```python
from build123d import *

# Parameters (mm, degrees)
SALIENTE_EXTRUIR2_DEPTH = 24
CROQUIS2_W              = 4.5
CROQUIS2_H              = 8
SALIENTE_EXTRUIR3_DEPTH = 24
CROQUIS3_W              = 7.5
CROQUIS3_H              = 3
SALIENTE_EXTRUIR4_DEPTH = 24
CORTAR_EXTRUIR1_START   = -8.720486
CROQUIS4_R              = 1.75
CORTAR_EXTRUIR1_DEPTH   = 17.440972
CROQUIS5_R              = 1.75
CORTAR_EXTRUIR2_DEPTH   = 10


with BuildPart() as part:
    # Croquis1 → Saliente-Extruir2 (new body)
    with BuildSketch(Plane.XY):
        with BuildLine():
            Line((-4.220485754, 10), (-12.5, 10))
            Line((-12.5, 10), (-12.5, -10))
            Line((-12.5, -10), (12.5, -10))
            Line((12.5, -10), (12.5, 10))
            Line((12.5, 10), (4.220485754, 10))
            ThreePointArc((4.220485754, 10), (0, -4.25), (-4.220485754, 10))
        make_face()
    extrude(amount=SALIENTE_EXTRUIR2_DEPTH)

    # Croquis2 → Saliente-Extruir3 (add)
    with BuildSketch(Plane.XY):
        with Locations((-6.470485754, 14)):
            Rectangle(CROQUIS2_W, CROQUIS2_H)
        with Locations((6.470485754, 14)):
            Rectangle(CROQUIS2_W, CROQUIS2_H)
    extrude(amount=SALIENTE_EXTRUIR3_DEPTH)

    # Croquis3 → Saliente-Extruir4 (add)
    with BuildSketch(Plane.XY):
        with Locations((-16.25, -8.5)):
            Rectangle(CROQUIS3_W, CROQUIS3_H)
        with Locations((16.25, -8.5)):
            Rectangle(CROQUIS3_W, CROQUIS3_H)
    extrude(amount=SALIENTE_EXTRUIR4_DEPTH)

    # Croquis4 → Cortar-Extruir1 (cut)
    with BuildSketch(Plane(origin=(0, 0, 0), x_dir=(0, 0, -1), z_dir=(1, 0, 0)).offset(CORTAR_EXTRUIR1_START)):
        with Locations((-20.5, 15)):
            Circle(CROQUIS4_R)
        with Locations((-12, 15)):
            Circle(CROQUIS4_R)
        with Locations((-3.5, 15)):
            Circle(CROQUIS4_R)
    extrude(amount=CORTAR_EXTRUIR1_DEPTH, mode=Mode.SUBTRACT)

    # Croquis5 → Cortar-Extruir2 (cut)
    with BuildSketch(Plane(origin=(0, 0, 0), x_dir=(1, 0, 0), z_dir=(0, 1, 0))):
        with Locations((-16.25, -12)):
            Circle(CROQUIS5_R)
        with Locations((16.25, -12)):
            Circle(CROQUIS5_R)
    extrude(amount=-CORTAR_EXTRUIR2_DEPTH, mode=Mode.SUBTRACT)


solid = part.part
```
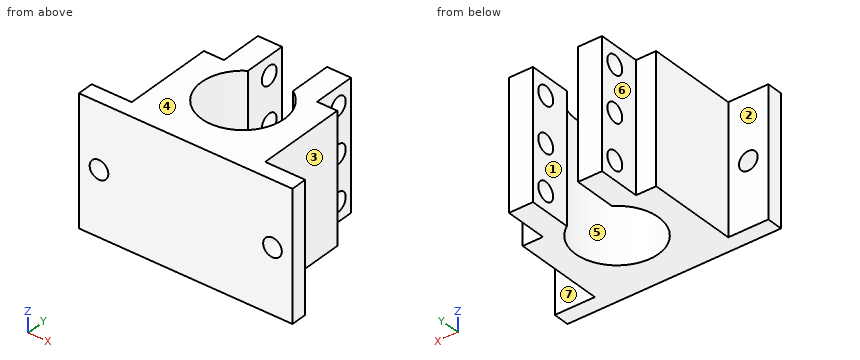
Here's how the part is built. I have some questions about the finished solid (model axes, mm). Face numbers are marked on the shaded views. A direction names the side the tool comes from. Coordinates: 2 decimals unless noted, no trailing zeros. Write each loop counter-clockwise with the first axis right and the second up, starting at its lowest first coordinate (ties: lowest second). Pieces come first, ordered by that corner, then holes. Notation, with made-up numbers: M 40.25,70 L 47.25,70 A14 cw 47.25,77 Z; hole C 60.25,-24 d8. An arc over 180 degrees is marked long. Answer as CSV lines item,"result". Start each with the question number.
Q1. If we mould it in two halves opening along X, with no side actions, what happens to the marked faces 5, 6 and 7? For each: pulls with the +X half, pulls with the -X half, needs draft (parallel to the pull), parting line crosses it, or undercut.
Q2. Suppose I cut it at B-B, the plane x = -16.25. List the corners of the cut face in (y, z) for me, then the cut area to 3 significant figures.
Q3. Suppose I cut it at A-A, the plane y = 3.5. List the corners of the cut face in (x, z) for me.
Q4. I need wall thicknesses on probe 1 along Z at (x, y) = (6.9, 15); probe 2 along X at (y, z) = (-7.9, 12); probe 3 along Y at (x, z) = (-5.35, 20.5). Which ranges of each line are inside material? Lowest first, please. Write a range as [from, to].
Q5. Will these pins go through, and if not, where does the flat tip stop? pin 1 Ø5.5 at (y, z) = (15, 12) entering from -X; pin 2 Ø10 at (y, z) = (5, 3) entering from -X; pin 3 Ø5.5 at (x, z) = (16.25, 12) entering from +Y; pin 4 Ø3 at (x, z) = (-16.25, 12) entering from -Y.
Q6. Suppose I cut it at C-C, the plane y = 15. State how many separate pieces and enclosed holes the cut face has, then the cut area to 4 significant figures.
Q7. For the marked faces 1, 2, 3 and 4, which set-ups out of +Z, -Z, +X, -X, +Y, -Y let a thin tool reach every point of the face, with its end or its side?
Q8. Suppose I cut it at D-D, the plane z = 4.75. List the corners of the cut face in (x, y) for me, then the cut area to 3 significant figures.
Entries:
1,face 5,"undercut"
1,face 6,"pulls with the -X half"
1,face 7,"needs draft"
2,outline,"M -10,0 L -7,0 L -7,10.25 L -10,10.25 Z; M -10,13.75 L -7,13.75 L -7,24 L -10,24 Z"
2,area,"61.5 mm²"
3,outline,"M -12.5,0 L -7.75,0 L -7.75,24 L -12.5,24 Z; M 7.75,0 L 12.5,0 L 12.5,24 L 7.75,24 Z"
4,probe 1,"z = [0, 1.75], [5.25, 10.25], [13.75, 18.75], [22.25, 24]"
4,probe 2,"x = [-20, -18], [-14.5, 14.5], [18, 20]"
4,probe 3,"y = [-10, -2.11], [9.11, 13.25], [16.75, 18]"
5,pin 1,"stops at x = -8.72"
5,pin 2,"stops at x = -12.5"
5,pin 3,"stops at y = -7"
5,pin 4,"passes through"
6,separate pieces,"8"
6,enclosed holes,"0"
6,area,"121.5 mm²"
7,face 1,"+Z, -Z, +Y"
7,face 2,"+Z, -Z, -X, +Y"
7,face 3,"+Z, -Z, +X, +Y"
7,face 4,"+Z, +X, -X, +Y, -Y"
8,outline,"M -20,-10 L 20,-10 L 20,-7 L 12.5,-7 L 12.5,10 L 8.72,10 L 8.72,13.78 L 4.22,13.78 L 4.22,10 A7.75 cw long -4.22,10 L -4.22,13.78 L -8.72,13.78 L -8.72,10 L -12.5,10 L -12.5,-7 L -20,-7 Z; M -8.72,16.22 L -4.22,16.22 L -4.22,18 L -8.72,18 Z; M 4.22,16.22 L 8.72,16.22 L 8.72,18 L 4.22,18 Z"
8,area,"413 mm²"
